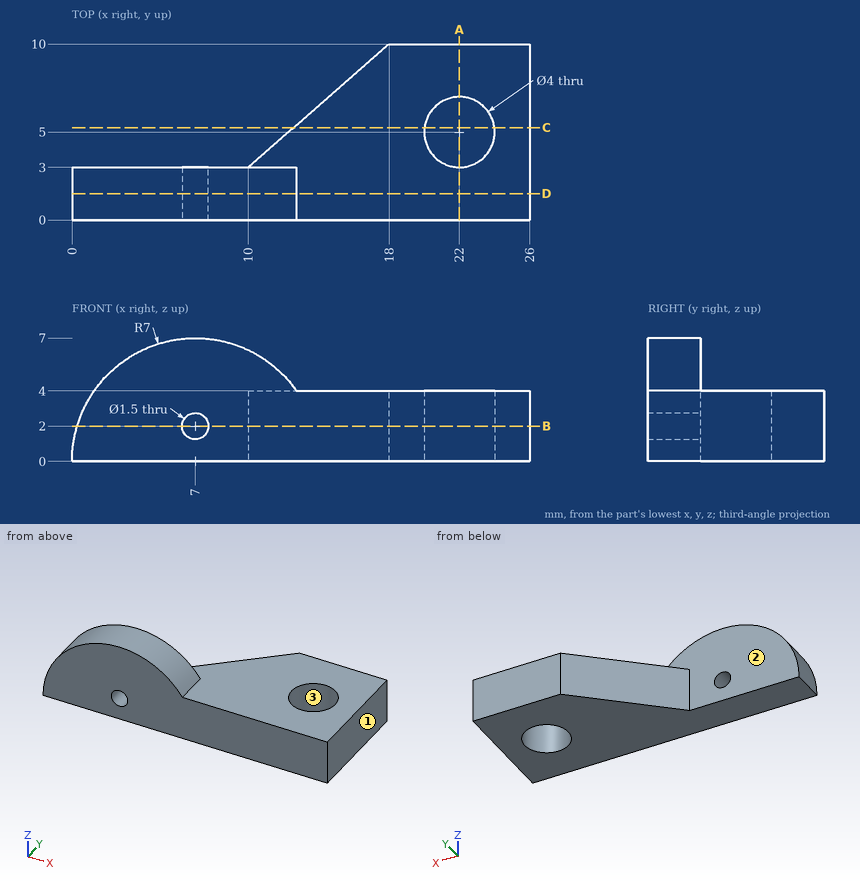
The figure shows three views and two pictorial views of one solid part (mm, origin at its lowest corner). Answer the questions. Round coordinates to 2 decimals unless told otherwise and drop trailing zeros. Order: outer loops, then holes, each group sorted by start corner. A loop starts at its lowest first (then second) coordinate and runs counter-clockwise, first axis right, second up. Notation, with made-up numbers: M -8.5,49.25 L 21.5,49.25 A22 ccw 21.5,76.25 Z; hole C 27,-11.75 d11. An arc over 180 degrees is marked long. Answer in a Markdown table with one row per item. Add a question column.
1) Flat-ended cylindrical pins translate along their axes: pin 1 Ø2.5 at (x, z) = (7, 2) entering from +Y; pin 2 Ø5 at (x, y) = (11, 1.5) entering from +Z; pin 3 Ø4 at (x, y) = (6.5, 4) entering from -Z; pin 4 Ø2 at (y, z) = (6, 1) entering from -X. Find the tip coordinate at first contact, or state that the pin passes through.
2) The part is cut by section B-B on z = 2. Determine the outline of the cut face in (x, y).
3) The part is cut by section D-D on y = 1.5. Determine the outline of the cut face in (x, z).
4) Determine the mould class of the marked faces 1, 2 and 3 for opening direction Y: pulls with the +Y half, pulls with the -Y half, needs draft (parallel to the pull), parting line crosses it, or undercut.
5) The part is cut by section C-C on y = 5.25. Determine the outline of the cut face in (x, z).
6) Consider line 1 along Y through (x, z) = (22, 2.3); line 2 along Z through (x, y) = (7, 2.05); line 3 along Z through (x, y) = (18.25, 1.5). Determine where each line is inside the solid, lowest interval first. Write a range as from..to.
7) The part is cut by section A-A on x = 22. Determine the outline of the cut face in (y, z), plus the area to 3 significant figures.
Findings below:
| question | item | result |
|---|---|---|
| 1 | pin 1 | stops at y = 3 |
| 1 | pin 2 | stops at z = 6.84 |
| 1 | pin 3 | stops at z = 0 |
| 1 | pin 4 | stops at x = 12.29 |
| 2 | outline | M 0.29,0 L 6.25,0 L 6.25,3 L 0.29,3 Z; M 7.75,0 L 26,0 L 26,10 L 18,10 L 10,3 L 7.75,3 Z; hole C 22,5 d4 |
| 3 | outline | M 0,0 L 26,0 L 26,4 L 12.74,4 A7 ccw Z; hole C 7,2 d1.5 |
| 4 | face 1 | needs draft |
| 4 | face 2 | pulls with the +Y half |
| 4 | face 3 | undercut |
| 5 | outline | M 12.57,0 L 20.02,0 L 20.02,4 L 12.57,4 Z; M 23.98,0 L 26,0 L 26,4 L 23.98,4 Z |
| 6 | line 1 | y = 0..3, 7..10 |
| 6 | line 2 | z = 0..1.25, 2.75..7 |
| 6 | line 3 | z = 0..4 |
| 7 | outline | M 0,0 L 3,0 L 3,4 L 0,4 Z; M 7,0 L 10,0 L 10,4 L 7,4 Z |
| 7 | area | 24.0 mm² |
